```python
from build123d import *

# Parameters (mm, degrees)
F0_R     = 38.1
F1_DEPTH = 76.2
F4_R     = 6.3246
F6_R     = 32.1196500774
F7_DEPTH = 50.038
F8_R     = 5.08
F9_R     = 6.35


with BuildPart() as f1:
    # F0 (on Top) → F1 (new body)
    with BuildSketch(Plane.XY):
        Circle(F0_R)
    extrude(amount=F1_DEPTH)

    # F5: sweep along a path in F2
    with BuildLine(Plane.XZ) as f5_path:
        ThreePointArc((33.5242934525, 16.8796218932), (70.7589105159, 39.7583444109), (32.8120825502, 61.4353114321))
    # F4 (on offset) → F5 (sweep)
    with BuildSketch(Plane.YZ.offset(37.846)):
        with Locations((0, 63.6169761419)):
            Circle(F4_R)
    sweep(path=f5_path.line)

    # F6 (on face) → F7 (cut)
    with BuildSketch(Plane.XY.offset(76.2)):
        Circle(F6_R)
    extrude(amount=-F7_DEPTH, mode=Mode.SUBTRACT)

    # F8
    f8_edges = [f1.edges().sort_by_distance(p)[0] for p in [
        (-38.1, 0, 76.2),
    ]]
    fillet(f8_edges, radius=F8_R)

    # F9
    f9_edges = [f1.edges().sort_by_distance(p)[0] for p in [
        (-38.1, 0, 0),
    ]]
    fillet(f9_edges, radius=F9_R)


solid = f1.part
```
Source: CAD feature listing. Evaluate the final solid. Frame: model axes, mm. A direction names the side the tool comes from. Round coordinates to 2 decimals unless told otherwise and drop trailing zeros. Loops run counter-clockwise (first coordinate to the right, second up) from the corner with the lowest first, then second, coordinate; pieces in that order, holes last.
1. Mould query, pull axis X, two halves, no side actions, for faces 3 (the cylindrical face through (-25.49, -19.54, 51.53)), 4 (the flat face through (0, 0, 0)). Classes: released by +X, released by -X, zero draft, split by the parting line, or undercut.
2. Contact query for flat-ended pins moving along their axis: pin 1 (8 mm diameter, centred on y = -19, z = 62, fed in from +X); pin 2 (19.5 mm diameter, centred on x = 5, y = -10, fed in from +Z); pin 3 (1 mm diameter, centred on y = 27.5, z = 45.5, fed in from -X); pin 4 (10 mm diameter, centred on x = 25, y = -3, fed in from -Z). Output: stop coordinate, or through.
3. Access query for faces 1 (the flat face through (7, -32, 76.2)), 2 (the flat face through (0, 0, 26.162)). Directions: +Z, -Z, +X, -X, +Y, -Y. A direction counts if a zero-diameter tool reaches every point of the face in a straight line with its end or side. Return the directions, or none.
4. Ray query, L1, parallel to Y at x = 0, z = 57; L2, parallel to Z at x = -11, y = 7; L3, parallel to X at y = -0.5, z = 46.5. Return the intervals inside material, ascending.
5. Section query B-B on z = 29. Give the number of separate pieces and of enclosed holes in the cut face, and give its area (3 significant figures).
6. Section query A-A on x = 0. Output: boundary loops of the cut face in (y, z).
Answers below:
1. face 3: undercut
1. face 4: zero draft
2. pin 1: stops at x = 35.02
2. pin 2: stops at z = 26.16
2. pin 3: stops at x = -26.88
2. pin 4: stops at z = 0
3. face 1: +Z, +X, -X, +Y, -Y
3. face 2: +Z
4. L1: y = -38.1 to -32.12, 32.12 to 38.1
4. L2: z = 0 to 26.16
4. L3: x = -38.1 to -32.12, 32.12 to 38.1, 63.47 to 76.02
5. separate pieces: 2
5. enclosed holes: 1
5. area: 1,450 mm2
6. outline: (-38.1, 6.35) arc R6.35 ccw to (-31.75, 0) - (31.75, 0) arc R6.35 ccw to (38.1, 6.35) - (38.1, 71.12) arc R5.08 ccw to (33.02, 76.2) - (32.12, 76.2) - (32.12, 26.16) - (-32.12, 26.16) - (-32.12, 76.2) - (-33.02, 76.2) arc R5.08 ccw to (-38.1, 71.12) - close
